from build123d import *

# Parameters (mm, degrees)
SKETCH11_W     = 187.05178758
SKETCH11_H     = 103.91050065
EXTRUDE3_DEPTH = 19.05
SKETCH12_W     = 187.05178758
SKETCH12_H     = 103.91050065
EXTRUDE4_DEPTH = 3.175


with BuildPart() as part:
    # Sketch11 → Extrude3 (new body)
    with BuildSketch(Plane(origin=(0, 0, 0), x_dir=(1, 0, 0), z_dir=(0, 1, 0))):
        with Locations((93.52589379, 51.955250325)):
            Rectangle(SKETCH11_W, SKETCH11_H)
        with BuildLine():
            Line((9.525, 6.35), (116.541319734, 6.35))
            ThreePointArc((116.541319734, 6.35), (118.786383764, 7.27993597), (119.716319734, 9.525))
            Line((119.716319734, 9.525), (119.716319734, 94.38550065))
            ThreePointArc((119.716319734, 94.38550065), (118.786383764, 96.63056468), (116.541319734, 97.56050065))
            Line((116.541319734, 97.56050065), (9.525, 97.56050065))
            ThreePointArc((9.525, 97.56050065), (7.27993597, 96.63056468), (6.35, 94.38550065))
            Line((6.35, 94.38550065), (6.35, 9.525))
            ThreePointArc((6.35, 9.525), (7.27993597, 7.27993597), (9.525, 6.35))
        make_face(mode=Mode.SUBTRACT)
        with BuildLine():
            Line((180.70178758, 9.525), (180.70178758, 94.38550065))
            ThreePointArc((180.70178758, 94.38550065), (179.77185161, 96.63056468), (177.52678758, 97.56050065))
            Line((177.52678758, 97.56050065), (129.241319734, 97.56050065))
            ThreePointArc((129.241319734, 97.56050065), (126.996255703, 96.63056468), (126.066319734, 94.38550065))
            Line((126.066319734, 94.38550065), (126.066319734, 9.525))
            ThreePointArc((126.066319734, 9.525), (126.996255703, 7.27993597), (129.241319734, 6.35))
            Line((129.241319734, 6.35), (177.52678758, 6.35))
            ThreePointArc((177.52678758, 6.35), (179.77185161, 7.27993597), (180.70178758, 9.525))
        make_face(mode=Mode.SUBTRACT)
    extrude(amount=EXTRUDE3_DEPTH)

    # Sketch12 → Extrude4 (add)
    with BuildSketch(Plane(origin=(0, 0, 0), x_dir=(1, 0, 0), z_dir=(0, 1, 0))):
        with Locations((93.52589379, 51.955250325)):
            Rectangle(SKETCH12_W, SKETCH12_H)
    extrude(amount=-EXTRUDE4_DEPTH)


solid = part.part
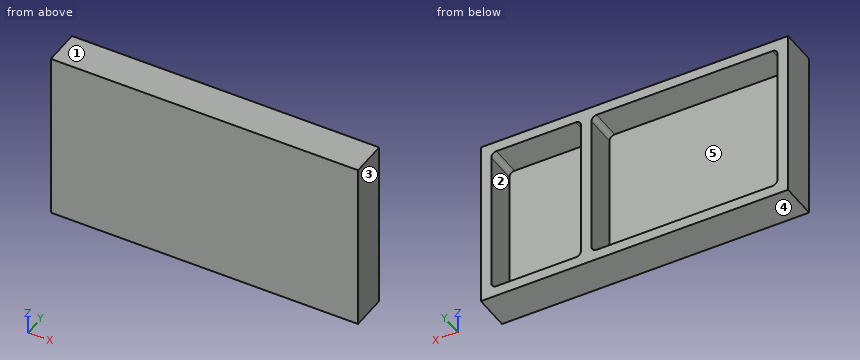
Geometry check sheet. Reference: the model listing, model coordinates, mm. Face numbers are marked on the shaded views. A direction names the side the tool comes from. Round coordinates to 2 decimals unless told otherwise and drop trailing zeros. Write each loop counter-clockwise with the first axis right and the second up, starting at its lowest first coordinate (ties: lowest second). Pieces come first, ordered by that corner, then holes.
Item 1: Access from +Z, -Z, +X, -X, +Y, -Y to the whole of each face (thin tool, end or side, straight path). Record for the marked faces 4 and 5.
Determined:
face 4: -Z, +X, -X, +Y, -Y
face 5: +Y
Item 2: Mould release check, pull along Z, two halves, no side actions. Record for the marked faces 1, 2 and 3: +Z half, -Z half, draft (parallel to the pull), parting line (faces both ways), or undercut.
Determined:
face 1: +Z half
face 2: undercut
face 3: draft
Item 3: Section check C-C (z = -14.5). Record the boundary of the cut face in (x, y) (3 decimals), plus the area to 3 significant figures.
Determined:
outline: (0, -3.175) - (187.052, -3.175) - (187.052, 19.05) - (180.702, 19.05) - (180.702, 0) - (126.066, 0) - (126.066, 19.05) - (119.716, 19.05) - (119.716, 0) - (6.35, 0) - (6.35, 19.05) - (0, 19.05) - close
area: 957 mm2
Item 4: Section check A-A (y = 11.75). Give the number of separate pieces and of enclosed holes in the cut face, plus the area to 3 significant figures.
Determined:
separate pieces: 1
enclosed holes: 2
area: 4,130 mm2
Item 5: Go/stop test with a flat-tipped pin: pin 1 Ø10 at (x, z) = (19.5, -30) entering from +Y. Record where the tip stops, or that it passes through.
Determined:
pin 1: stops at y = 0
Item 6: Material ranges on line 1 along X through (y, z) = (12.75, -34.5); line 2 along Z through (x, y) = (159.5, 13.25), recorded low to high.
Determined:
line 1: x = 0 to 6.35, 119.72 to 126.07, 180.7 to 187.05
line 2: z = -103.91 to -97.56, -6.35 to 0
